from build123d import *

# Parameters (mm, degrees)
BASE_FLANGE1_DEPTH      = 45
EDGE_FLANGE2_START      = -100
EDGE_FLANGE2_DEPTH      = 200
EDGE_FLANGE2_2_DEPTH    = 4
EDGE_FLANGE2_START_2    = 96
EDGE_FLANGE2_3_DEPTH    = 4
EDGE_FLANGE2_START_3    = -96
EDGE_FLANGE2_4_DEPTH    = 192
EDGE_FLANGE3_START      = -100
EDGE_FLANGE3_DEPTH      = 200
EDGE_FLANGE3_2_DEPTH    = 4
EDGE_FLANGE3_START_2    = 96
EDGE_FLANGE3_3_DEPTH    = 4
EDGE_FLANGE3_START_3    = -96
EDGE_FLANGE3_4_DEPTH    = 192
CUT_EXTRUDE1_DEPTH      = 121.519707932
CUT_EXTRUDE1_DEPTH_BACK = 121.519707932
CUT_EXTRUDE2_DEPTH      = 138.840487521
CUT_EXTRUDE2_DEPTH_BACK = 45
EDGE_FLANGE4_DEPTH      = 36
FILLET1_R               = 5
CUT_EXTRUDE3_DEPTH      = 10


# Read off the part's stored shape, not the designer's step: Edge-Flange2, Edge-Flange3
# Sheet-metal steps are written as plain solids
with BuildPart() as part:
    # Sketch1 → Base-Flange1 (new, symmetric)
    with BuildSketch(Plane.XY):
        with BuildLine():
            Line((-100, 0), (-100, 26))
            ThreePointArc((-100, 26), (-98.828427125, 28.828427125), (-96, 30))
            Line((-96, 30), (96, 30))
            ThreePointArc((96, 30), (98.828427125, 28.828427125), (100, 26))
            Line((100, 26), (100, 0))
            Line((100, 0), (98, 0))
            Line((98, 0), (98, 26))
            ThreePointArc((98, 26), (97.414213562, 27.414213562), (96, 28))
            Line((96, 28), (-96, 28))
            ThreePointArc((-96, 28), (-97.414213562, 27.414213562), (-98, 26))
            Line((-98, 26), (-98, 0))
            Line((-98, 0), (-100, 0))
        make_face()
    extrude(amount=BASE_FLANGE1_DEPTH, both=True)

    # Edge-Flange2 outline → Edge-Flange2 (cut)
    with BuildSketch(Plane.YZ.offset(EDGE_FLANGE2_START)):
        with BuildLine():
            Line((26, 43), (26, 41))
            Line((26, 41), (28, 41))
            ThreePointArc((28, 41), (27.414213562, 42.414213562), (26, 43))
        make_face()
        with BuildLine():
            ThreePointArc((26, 45), (28.828427125, 43.828427125), (30, 41))
            Line((30, 41), (30, 45))
            Line((30, 45), (26, 45))
        make_face()
    extrude(amount=EDGE_FLANGE2_DEPTH, mode=Mode.SUBTRACT)

    # Edge-Flange2 2 outline → Edge-Flange2 2 (cut)
    with BuildSketch(Plane.YZ.offset(EDGE_FLANGE2_START)):
        with BuildLine():
            Line((26, 45), (26, 43))
            ThreePointArc((26, 43), (27.414213562, 42.414213562), (28, 41))
            Line((28, 41), (30, 41))
            ThreePointArc((30, 41), (28.828427125, 43.828427125), (26, 45))
        make_face()
    extrude(amount=EDGE_FLANGE2_2_DEPTH, mode=Mode.SUBTRACT)

    # Edge-Flange2 3 outline → Edge-Flange2 3 (cut)
    with BuildSketch(Plane.YZ.offset(EDGE_FLANGE2_START_2)):
        with BuildLine():
            Line((26, 45), (26, 43))
            ThreePointArc((26, 43), (27.414213562, 42.414213562), (28, 41))
            Line((28, 41), (30, 41))
            ThreePointArc((30, 41), (28.828427125, 43.828427125), (26, 45))
        make_face()
    extrude(amount=EDGE_FLANGE2_3_DEPTH, mode=Mode.SUBTRACT)

    # Edge-Flange2 4 outline → Edge-Flange2 4 (add)
    with BuildSketch(Plane.YZ.offset(EDGE_FLANGE2_START_3)):
        with BuildLine():
            Line((-20, 43), (26, 43))
            ThreePointArc((26, 43), (27.414213562, 42.414213562), (28, 41))
            Line((28, 41), (28, 44.464101616))
            ThreePointArc((28, 44.464101616), (27.03527618, 44.863703305), (26, 45))
            Line((26, 45), (-20, 45))
            Line((-20, 45), (-20, 43))
        make_face()
    extrude(amount=EDGE_FLANGE2_4_DEPTH)

    # Edge-Flange3 outline → Edge-Flange3 (cut)
    with BuildSketch(Plane.YZ.offset(EDGE_FLANGE3_START)):
        with BuildLine():
            Line((28, -41), (26, -41))
            Line((26, -41), (26, -43))
            ThreePointArc((26, -43), (27.414213562, -42.414213562), (28, -41))
        make_face()
        with BuildLine():
            Line((26, -45), (30, -45))
            Line((30, -45), (30, -41))
            ThreePointArc((30, -41), (28.828427125, -43.828427125), (26, -45))
        make_face()
    extrude(amount=EDGE_FLANGE3_DEPTH, mode=Mode.SUBTRACT)

    # Edge-Flange3 2 outline → Edge-Flange3 2 (cut)
    with BuildSketch(Plane.YZ.offset(EDGE_FLANGE3_START)):
        with BuildLine():
            ThreePointArc((28, -41), (27.414213562, -42.414213562), (26, -43))
            Line((26, -43), (26, -45))
            ThreePointArc((26, -45), (28.828427125, -43.828427125), (30, -41))
            Line((30, -41), (28, -41))
        make_face()
    extrude(amount=EDGE_FLANGE3_2_DEPTH, mode=Mode.SUBTRACT)

    # Edge-Flange3 3 outline → Edge-Flange3 3 (cut)
    with BuildSketch(Plane.YZ.offset(EDGE_FLANGE3_START_2)):
        with BuildLine():
            ThreePointArc((28, -41), (27.414213562, -42.414213562), (26, -43))
            Line((26, -43), (26, -45))
            ThreePointArc((26, -45), (28.828427125, -43.828427125), (30, -41))
            Line((30, -41), (28, -41))
        make_face()
    extrude(amount=EDGE_FLANGE3_3_DEPTH, mode=Mode.SUBTRACT)

    # Edge-Flange3 4 outline → Edge-Flange3 4 (add)
    with BuildSketch(Plane.YZ.offset(EDGE_FLANGE3_START_3)):
        with BuildLine():
            ThreePointArc((28, -41), (27.414213562, -42.414213562), (26, -43))
            Line((26, -43), (-20, -43))
            Line((-20, -43), (-20, -45))
            Line((-20, -45), (26, -45))
            ThreePointArc((26, -45), (27.03527618, -44.863703305), (28, -44.464101616))
            Line((28, -44.464101616), (28, -41))
        make_face()
    extrude(amount=EDGE_FLANGE3_4_DEPTH)

    # Sketch15 → Cut-Extrude1 (cut, two sides: drawn at the far end of the back side and taken through both)
    with BuildSketch(Plane(origin=(0, 30, 0), x_dir=(1, 0, 0), z_dir=(0, 1, 0)).offset(-CUT_EXTRUDE1_DEPTH_BACK)):
        with BuildLine():
            Line((-60, 65.269806107), (-60, 25))
            ThreePointArc((-60, 25), (-61.464466094, 21.464466094), (-65, 20))
            Line((-65, 20), (-105.792448389, 20))
            Line((-105.792448389, 20), (-105.792448389, 65.269806107))
            Line((-105.792448389, 65.269806107), (-60, 65.269806107))
        make_face()
        with BuildLine():
            Line((105.792448389, 65.269806107), (60, 65.269806107))
            Line((60, 65.269806107), (60, 25))
            ThreePointArc((60, 25), (61.464466094, 21.464466094), (65, 20))
            Line((65, 20), (105.792448389, 20))
            Line((105.792448389, 20), (105.792448389, 65.269806107))
        make_face()
        with BuildLine():
            Line((60, -65.269806107), (60, -25))
            ThreePointArc((60, -25), (61.464466094, -21.464466094), (65, -20))
            Line((65, -20), (105.792448389, -20))
            Line((105.792448389, -20), (105.792448389, -65.269806107))
            Line((105.792448389, -65.269806107), (60, -65.269806107))
        make_face()
        with BuildLine():
            Line((-105.792448389, -20), (-105.792448389, -65.269806107))
            Line((-105.792448389, -65.269806107), (-60, -65.269806107))
            Line((-60, -65.269806107), (-60, -25))
            ThreePointArc((-60, -25), (-61.464466094, -21.464466094), (-65, -20))
            Line((-65, -20), (-105.792448389, -20))
        make_face()
    extrude(amount=CUT_EXTRUDE1_DEPTH + CUT_EXTRUDE1_DEPTH_BACK, mode=Mode.SUBTRACT)

    # Sketch16 → Cut-Extrude2 (cut, two sides: drawn at the far end of the back side and taken through both)
    with BuildSketch(Plane.XY.offset(45).offset(-CUT_EXTRUDE2_DEPTH_BACK)):
        with BuildLine():
            Line((0, 30), (0, 6.71))
            ThreePointArc((0, 6.71), (1.464466094, 3.174466094), (5, 1.71))
            Line((5, 1.71), (25, 1.71))
            ThreePointArc((25, 1.71), (28.535533906, 3.174466094), (30, 6.71))
            Line((30, 6.71), (30, 30))
            Line((30, 30), (0, 30))
        make_face()
    extrude(amount=CUT_EXTRUDE2_DEPTH + CUT_EXTRUDE2_DEPTH_BACK, mode=Mode.SUBTRACT)

    # Edge-Flange4 section (across the edge) → Edge-Flange4 (add)
    with BuildSketch(Plane(origin=(2, 30, 41), x_dir=(-1, 0, 0), z_dir=(0, 0, -1))):
        with BuildLine():
            Line((-2, 2), (-2, 18))
            Line((-2, 18), (0, 18))
            Line((0, 18), (0, 2))
            ThreePointArc((0, 2), (0.585786438, 0.585786438), (2, 0))
            Line((2, 0), (2, -2))
            ThreePointArc((2, -2), (-0.828427125, -0.828427125), (-2, 2))
        make_face()
    extrude(amount=EDGE_FLANGE4_DEPTH)

    # Fillet1
    fillet1_edges = [part.edges().sort_by_distance(p)[0] for p in [
        (3, 48, 5),
        (3, 48, 41),
        (-99, 0, 20),
        (-60, -20, 44),
        (60, -20, 44),
        (99, 0, -20),
        (-60, -20, -44),
        (-99, 0, -20),
        (99, 0, 20),
        (60, -20, -44),
        (0, 29, 0),
        (30, 29, 0),
    ]]
    fillet(fillet1_edges, radius=FILLET1_R - 0.0001)  # a hair under: the kernel refuses the full size

    # Sketch21 → Cut-Extrude3 (cut)
    with BuildSketch(Plane.ZY.offset(-2)):
        with BuildLine():
            Line((18, 43.5), (28, 43.5))
            ThreePointArc((28, 43.5), (31.5, 40), (28, 36.5))
            Line((28, 36.5), (18, 36.5))
            ThreePointArc((18, 36.5), (14.5, 40), (18, 43.5))
        make_face()
    extrude(amount=-CUT_EXTRUDE3_DEPTH, mode=Mode.SUBTRACT)


solid = part.part
Model file for the job. Use its own axes, mm. A direction names the side the tool comes from. Give positions to 0.01 mm unless a question says otherwise; leave off trailing zeros. Order: outer loops, then holes, each group sorted by start corner. A loop starts at its lowest first (then second) coordinate and runs counter-clockwise, first axis right, second up. Notation, with made-up numbers: (76.5, -7) - (105.5, -7) arc R5 cw to (105.5, 0) - close; hole circle Ø10 at (45, -26.75). An arc over 180 degrees is marked (long way). Write item = value, one per line. Start each with the question number.
1. Cut at B-B, the plane x = 7. List the corners of the cut face in (y, z), and give its area (3 significant figures).
2. Probe line 1 along Z through (x, y) = (39.5, 1); line 2 along X through (y, z) = (18, -4.5); line 3 along Y through (x, z) = (23.5, -15). List the from-to ranges inside material, lowest first.
3. Cut at C-C, the plane y = 40. List the corners of the cut face in (x, z), and give its area (3 significant figures).
4. Cut at D-D, the plane z = -9.5. List the corners of the cut face in (x, y).
5. Which spindle directions (+Z, -Z, +X, -X, +Y, -Y) get a long thin tool onto all of the face, cutting with end or side? Do faces 5 (the flat face through (-60, 12.4, 43.2)), 6 (the flat face through (-1, 3, 43)), 7 (the flat face through (0, 19, 44)). Say none if no direction does.
6. Two-plate mould, pull along X, no slides. Class faces 1 (the cylindrical face through (59, -18, -44)), 2 (the cylindrical face through (29, 29, 2)), 3 (the flat face through (-100, 13, 0)), 4 (the cylindrical face through (1, 29, 2)): pulls with the +X half, pulls with the -X half, needs draft (parallel to the pull), parting line crosses it, or undercut.
7. Cut at A-A, the plane y = 12.5. List the corners of the cut face in (x, z).
8. Drop flat-ended pins along their axis: P1, Ø1, axis at x = 12.5, z = 44.5, coming from the +Y side; P2, Ø3, axis at x = 2, y = 37.5, coming from the -Z side; P3, Ø4, axis at x = -73.5, z = -16, coming from the +Y side; P4, Ø16, axis at y = 6, z = 34.5, coming from the -X side. Give the stop position or say it passes through.
Taken from the geometry:
q1.outline = (-20, -45) - (26, -45) arc R4 ccw to (30, -41) - (30, 0) - (28, 0) - (28, -41) arc R2 cw to (26, -43) - (-20, -43) - close; (-20, 43) - (1.71, 43) - (1.71, 45) - (-20, 45) - close
q1.area = 227 mm²
q2.line_1 = -45 to -43, 43 to 45
q2.line_2 = -100 to -98, 98 to 100
q2.line_3 = 28 to 30
q3.outline = (2, 5) - (4, 5) - (4, 14.5) - (2, 14.5) - close; (2, 31.5) - (4, 31.5) - (4, 41) - (2, 41) - close
q3.area = 38.0 mm²
q4.outline = (-100, 0) - (-98, 0) - (-98, 26) arc R2 cw to (-96, 28) - (96, 28) arc R2 cw to (98, 26) - (98, 0) - (100, 0) - (100, 26) arc R4 ccw to (96, 30) - (-96, 30) arc R4 ccw to (-100, 26) - close
q5.face_5 = +Z, -X, +Y, -Y
q5.face_6 = +X, -X, -Y
q5.face_7 = +Z, +Y
q6.face_1 = pulls with the +X half
q6.face_2 = undercut
q6.face_3 = pulls with the -X half
q6.face_4 = undercut
q7.outline = (-100, -20) - (-98, -20) - (-98, 20) - (-100, 20) - close; (-60, -45) - (60, -45) - (60, -43) - (-60, -43) - close; (-60, 43) - (0, 43) - (0, 45) - (-60, 45) - close; (30, 43) - (60, 43) - (60, 45) - (30, 45) - close; (98, -20) - (100, -20) - (100, 20) - (98, 20) - close
q8.P1 = 1.71
q8.P2 = 5
q8.P3 = 30
q8.P4 = through
